Autodesk Inventor part; units mm, degrees
ref_plane "YZ Plane" through (0, 0, 0) normal (1, 0, 0) x (0, 1, 0)
ref_plane "XZ Plane" through (0, 0, 0) normal (0, 1, 0) x (-1, 0, 0)
ref_plane "XY Plane" through (0, 0, 0) normal (0, 0, 1) x (1, 0, 0)
sketch "Sketch1" plane through (0, 0, 0) normal (0, 1, 0) x (-1, 0, 0)
  circle A0 centre (0, 0) radius 177
  dimension "d0" = 354
extrude "Extrusion1" add sketch "Sketch1" along normal blind 4.7625
sketch "Sketch2" plane through (0, 4.7625, 0) normal (0, 1, 0) x (1, 0, 0)
  circle A0 centre (101.6, -101.6) radius 1.7
  circle A1 centre (101.6, 101.6) radius 1.7
  circle A2 centre (-101.6, 101.6) radius 1.7
  circle A3 centre (-101.6, -101.6) radius 1.7
  circle A4 centre (0, 0) radius 177
  dimension "d3" = 3.4
  dimension "d4" = 3.4
  dimension "d5" = 3.4
  dimension "d6" = 3.4
  dimension "d14" = 101.6
  dimension "d15" = 101.6
  dimension "d16" = 101.6
  dimension "d17" = 101.6
  dimension "d18" = 101.6
  dimension "d19" = 101.6
  dimension "d20" = 101.6
  dimension "d21" = 101.6
extrude "Standoff Holes" cut sketch "Sketch2" against normal through all contours A0 | A1 | A2 | A3
sketch "Sketch3" plane through (0, 4.7625, 0) normal (0, 1, 0) x (1, 0, 0)
  line L0 (-40, -144.3) -> (40, -144.3)
  line L1 (40, -144.3) -> (40, -114.3)
  line L2 (40, -114.3) -> (-40, -114.3)
  line L3 (-40, -114.3) -> (-40, -144.3)
  circle A0 centre (-25.4, -107.95) radius 1.7
  circle A1 centre (25.4, -107.95) radius 1.7
  circle A2 centre (25.4, -150.65) radius 1.7
  circle A3 centre (-25.4, -150.65) radius 1.7
  circle A4 centre (0, 0) radius 177
  line L4 (-177, 0) -> (177, 0)
  line L5 (-40, 144.3) -> (40, 144.3)
  line L6 (40, 144.3) -> (40, 114.3)
  line L7 (40, 114.3) -> (-40, 114.3)
  line L8 (-40, 114.3) -> (-40, 144.3)
  circle A5 centre (-25.4, 107.95) radius 1.7
  circle A6 centre (25.4, 107.95) radius 1.7
  circle A7 centre (25.4, 150.65) radius 1.7
  circle A8 centre (-25.4, 150.65) radius 1.7
  point P0 (0, -114.3)
  point P1 (0, 114.3)
  dimension "d25" = 80
  dimension "d26" = 30
  dimension "d28" = 114.3
  dimension "d30" = 40
  dimension "d32" = 3.4
  dimension "d33" = 3.4
  dimension "d34" = 3.4
  dimension "d35" = 3.4
  dimension "d36" = 6.35
  dimension "d37" = 6.35
  dimension "d38" = 6.35
  dimension "d39" = 6.35
  dimension "d40" = 25.4
  dimension "d41" = 25.4
  dimension "d42" = 25.4
  dimension "d43" = 25.4
  dimension "d44" = 228.6
extrude "Wheels" cut sketch "Sketch3" against normal blind 25.4 contours L3 L2 L1 L0 | A0 | A1 | A2 | A3 | L5 L6 L7 L8 | A5 | A6 | A7 | A8
sketch "Sketch4" plane through (0, 4.7625, 0) normal (0, 1, 0) x (1, 0, 0)
  circle A0 centre (13.4493, -63.76) radius 1.7
  circle A1 centre (13.4493, -21.9516) radius 1.7
  circle A2 centre (-13.4493, -63.76) radius 1.7
  circle A3 centre (-13.4493, -21.9516) radius 1.7
  line L0 (-40, -114.3) -> (40, -114.3)
  circle A4 centre (0, 0) radius 177
  line L1 (-177, 0) -> (177, 0) construction
  circle A5 centre (13.4493, 63.76) radius 1.7
  circle A6 centre (13.4493, 21.9516) radius 1.7
  circle A7 centre (-13.4493, 63.76) radius 1.7
  circle A8 centre (-13.4493, 21.9516) radius 1.7
  dimension "d47" = 3.4
  dimension "d48" = 3.4
  dimension "d49" = 3.4
  dimension "d50" = 3.4
  dimension "d51" = 26.8986
  dimension "d52" = 26.8986
  dimension "d53" = 41.8084
  dimension "d54" = 41.8084
  dimension "d55" = 13.4493
  dimension "d56" = 13.4493
  dimension "d57" = 50.54
  dimension "d84" = 13.4493
extrude "Motor Mount" cut sketch "Sketch4" against normal through all contours A0 | A1 | A2 | A3 | A5 | A6 | A7 | A8
sketch "Sketch5" plane through (0, 4.7625, 0) normal (0, 1, 0) x (1, 0, 0)
  circle A0 centre (-107.95, -53.7) radius 1.7
  circle A1 centre (-107.95, 38.8) radius 1.7
  circle A2 centre (-29.45, 38.8) radius 1.7
  circle A3 centre (-29.45, -53.7) radius 1.7
  point P0 (0, 0)
  dimension "d61" = 3.4
  dimension "d62" = 3.4
  dimension "d63" = 3.4
  dimension "d64" = 3.4
  dimension "d65" = 92.5
  dimension "d66" = 92.5
  dimension "d67" = 78.5
  dimension "d68" = 78.5
  dimension "d69" = 38.8
  dimension "d70" = 38.8
  dimension "d72" = 53.7
  dimension "d73" = 107.95
extrude "PCB" cut sketch "Sketch5" against normal blind 25.4
sketch "Sketch6" plane through (0, 4.7625, 0) normal (0, 1, 0) x (1, 0, 0)
  circle A0 centre (100.8, -20) radius 1.7
  circle A1 centre (100.8, 20) radius 1.7
  circle A2 centre (0, 0) radius 177
  line L0 (177, 0) -> (177, 59.2823) construction
  line L1 (0, -177) -> (0, 177) construction
  circle A3 centre (-100.8, -20) radius 1.7
  circle A4 centre (-100.8, 20) radius 1.7
  dimension "d76" = 3.4
  dimension "d77" = 3.4
  dimension "d78" = 40
  dimension "d80" = 20
  dimension "d81" = 76.2
  dimension "d98" = 100.8
extrude "Caster" cut sketch "Sketch6" against normal blind 25.4 contours A0 | A1 | A3 | A4
sketch "Sketch7" plane through (0, 4.7625, 0) normal (0, 1, 0) x (1, 0, 0)
  line L0 (-166.0395, -33.995) -> (-162.8645, -33.995)
  line L1 (-162.8645, -33.995) -> (-162.8645, -27.645)
  line L2 (-162.8645, -27.645) -> (-166.0395, -27.645)
  line L3 (-166.0395, -27.645) -> (-166.0395, -33.995)
  line L4 (-162.8645, -21.295) -> (-162.8645, -14.945)
  line L5 (-162.8645, -14.945) -> (-166.0395, -14.945)
  line L6 (-166.0395, -14.945) -> (-166.0395, -21.295)
  line L7 (-166.0395, -21.295) -> (-162.8645, -21.295)
  line L8 (-162.8645, -8.595) -> (-162.8645, -2.245)
  line L9 (-162.8645, -2.245) -> (-166.0395, -2.245)
  line L10 (-166.0395, -2.245) -> (-166.0395, -8.595)
  line L11 (-166.0395, -8.595) -> (-162.8645, -8.595)
  line L12 (-162.8645, 4.105) -> (-162.8645, 10.455)
  line L13 (-162.8645, 10.455) -> (-166.0395, 10.455)
  line L14 (-166.0395, 10.455) -> (-166.0395, 4.105)
  line L15 (-166.0395, 4.105) -> (-162.8645, 4.105)
  line L16 (-162.8645, 16.805) -> (-162.8645, 23.155)
  line L17 (-162.8645, 23.155) -> (-166.0395, 23.155)
  line L18 (-166.0395, 23.155) -> (-166.0395, 16.805)
  line L19 (-166.0395, 16.805) -> (-162.8645, 16.805)
  line L20 (-162.8645, 29.505) -> (-162.8645, 35.855)
  line L21 (-162.8645, 35.855) -> (-166.0395, 35.855)
  line L22 (-166.0395, 35.855) -> (-166.0395, 29.505)
  line L23 (-166.0395, 29.505) -> (-162.8645, 29.505)
  point P0 (0, 0)
  dimension "d85" = 6.35
  dimension "d86" = 3.175
  dimension "d89" = 12.7
  dimension "d94" = 162.8645
  dimension "d95" = 33.995
extrude "Switch" cut sketch "Sketch7" against normal through all
equation "\"d52\" = d51"
equation "\"d54\" = d53"
equation "\"d62\" = d61"
equation "\"d63\" = d61"
equation "\"d64\" = d61"
equation "\"d66\" = d65"
equation "\"d68\" = d67"
properties part number "layer1_narrow"
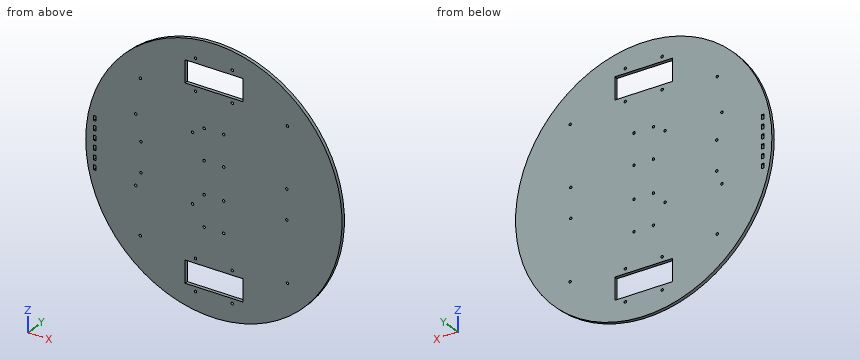
Part model, mm, in its own coordinate system. Round coordinates to 2 decimals unless told otherwise and drop trailing zeros. Order: outer loops, then holes, each group sorted by start corner. A loop starts at its lowest first (then second) coordinate and runs counter-clockwise, first axis right, second up. Notation, with made-up numbers: M -33,21.25 L 5,21.25 A14 cw 5,44.25 Z; hole C 79.25,0 d2. An arc over 180 degrees is marked long. Answer in a Markdown table with one row per item. Add a question column.
Q1. Pin check, flat tips, straight feed: pin 1 (2 mm diameter, centred on x = 101.6, z = -101.6, fed in from +Y) (1 decimal); pin 2 (2.5 mm diameter, centred on x = -165, y = 3.5, fed in from -Z); pin 3 (1.6 mm diameter, centred on x = -164, y = 1.5, fed in from +Z); pin 4 (1.6 mm diameter, centred on x = -165, y = 2.5, fed in from -Z). Stop position of each tip, or through.
Q2. Cut at A-A on x = -2.5. Give the cut face in (y, z).
Q3. Wall check: L1, parallel to X at y = 3, z = 101.6; L2, parallel to X at y = 1.6, z = -20; L3, parallel to Z at x = -100.8, y = 1.05. Give the ranges that are in metal, low to high. Write a range as from..to.
Q4. Cut at B-B on y = 1.85. Give the number of separate pieces and of enclosed holes in the cut face, and give its area (3 significant figures).
Established:
| question | item | result |
|---|---|---|
| 1 | pin 1 | passes through |
| 1 | pin 2 | stops at z = -67.19 |
| 1 | pin 3 | stops at z = 68.52 |
| 1 | pin 4 | stops at z = -66.09 |
| 2 | outline | M 0,-176.98 L 4.76,-176.98 L 4.76,-144.3 L 0,-144.3 Z; M 0,-114.3 L 4.76,-114.3 L 4.76,114.3 L 0,114.3 Z; M 0,144.3 L 4.76,144.3 L 4.76,176.98 L 0,176.98 Z |
| 3 | L1 | x = -144.94..-103.3, -99.9..99.9, 103.3..144.94 |
| 3 | L2 | x = -175.87..-166.04, -162.86..-102.5, -99.1..99.1, 102.5..175.87 |
| 3 | L3 | z = -145.49..-103.1, -100.1..-21.7, -18.3..18.3, 21.7..100.1, 103.1..145.49 |
| 4 | separate pieces | 1 |
| 4 | enclosed holes | 36 |
| 4 | area | 93,200 mm2 |
